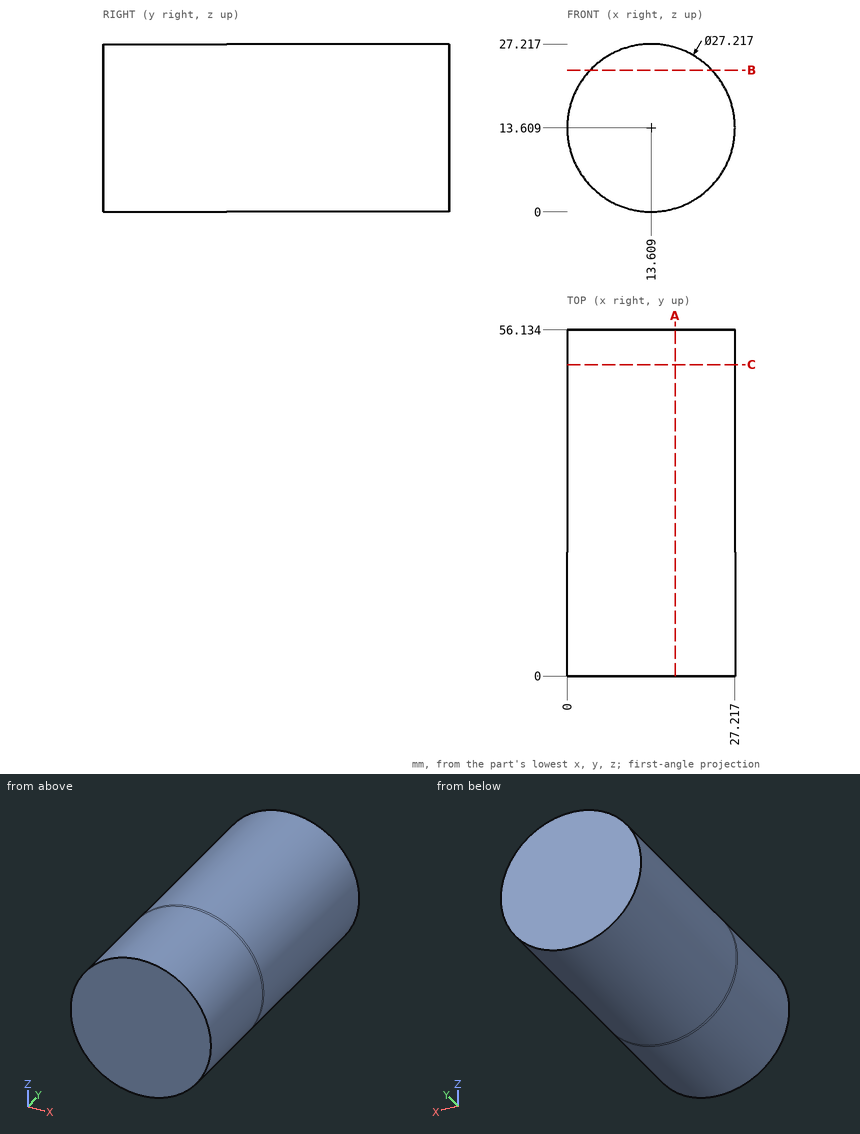
Input: dimensioned drawing with shaded views. Units: mm. Origin: part minimum x, y, z. Give positions to 0.01 mm unless a question says otherwise; leave off trailing zeros. Loops run counter-clockwise (first coordinate to the right, second up) from the corner with the lowest first, then second, coordinate; pieces in that order, holes last. Notation, with made-up numbers: (35.5, 64) - (82.5, 64) arc R22 ccw to (82.5, 73) - close; hole circle Ø7 at (-28.5, 2). An arc over 180 degrees is marked (long way). Answer as CSV lines item,"result". Start each with the question number.
(1) Ray query, line 1 along X through (y, z) = (26, 15.75); line 2 along X through (y, z) = (5.5, 3.5) (1 decimal); line 3 along Z through (x, y) = (2, 37.5) (1 decimal). Return the intervals inside material, ascending. Write a range as [from, to].
(2) Pin query (flat end, axial travel): P1, Ø1, axis at x = 4, y = 37, coming from the +Z side; P2, Ø5, axis at y = 16, z = 5, coming from the -X side; P3, Ø12, axis at x = 21.5, y = 43, coming from the -Z side. Return the tip coordinate at first contact, or that it passes through.
(3) Section query C-C (y = 50.5). Output: boundary loops of the cut face in (x, z).
(4) Section query B-B (z = 23). Output: boundary loops of the cut face in (x, y), and give its area (3 significant figures).
(5) Section query A-A (x = 17.5). Output: boundary loops of the cut face in (y, z), and give its area (3 significant figures).
Worked answers:
1,line 1,"x = [0.17, 27.05]"
1,line 2,"x = [4.5, 22.7]"
1,line 3,"z = [6.5, 20.7]"
2,P1,"stops at z = 23.72"
2,P2,"stops at x = 1.45"
2,P3,"stops at z = 0.13"
3,outline,"circle Ø27.22 at (13.61, 13.61)"
4,outline,"(3.76, 0) - (23.46, 0) - (23.46, 56.13) - (3.76, 56.13) - close"
4,area,"1,110 mm^2"
5,outline,"(0, 0.57) - (56.13, 0.57) - (56.13, 26.65) - (0, 26.65) - close"
5,area,"1,460 mm^2"
